```python
from build123d import *

# Parameters (mm, degrees)
F0_W     = 11.176
F0_H     = 26.5938
F1_DEPTH = 4.6482
F2_R     = 5.08
F4_DEPTH = 3.302


with BuildPart() as f1:
    # F0 (on Top) → F1 (new body)
    with BuildSketch(Plane.XY):
        Rectangle(F0_W, F0_H)
    extrude(amount=F1_DEPTH)

    # F2
    f2_edges = [f1.edges().sort_by_distance(p)[0] for p in [
        (-5.588, 13.2969, 2.3241),
        (5.588, 13.2969, 2.3241),
        (-5.588, -13.2969, 2.3241),
        (5.588, -13.2969, 2.3241),
    ]]
    fillet(f2_edges, radius=F2_R)

    # F3 (on face) → F4 (cut)
    with BuildSketch(Plane.XY):
        with BuildLine():
            Line((-4.938699, 8.085186), (-4.938699, -8.085186))
            ThreePointArc((-4.938699, -8.085186), (-3.599592, -11.318078), (-0.366699, -12.657186))
            Line((-0.366699, -12.657186), (0.366699, -12.657186))
            ThreePointArc((0.366699, -12.657186), (3.599592, -11.318078), (4.938699, -8.085186))
            Line((4.938699, -8.085186), (4.938699, 8.085186))
            ThreePointArc((4.938699, 8.085186), (3.599592, 11.318078), (0.366699, 12.657186))
            Line((0.366699, 12.657186), (-0.366699, 12.657186))
            ThreePointArc((-0.366699, 12.657186), (-3.599592, 11.318078), (-4.938699, 8.085186))
        make_face()
    extrude(amount=F4_DEPTH, mode=Mode.SUBTRACT)


solid = f1.part
```
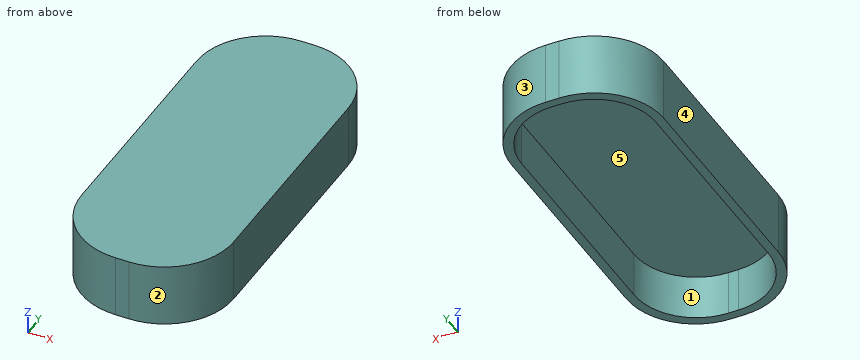
The model under review builds one solid part; all positions refer to its coordinate system, in mm. Face numbers are marked on the shaded views. A direction names the side the tool comes from. Round coordinates to 2 decimals unless told otherwise and drop trailing zeros. Order: outer loops, then holes, each group sorted by start corner. A loop starts at its lowest first (then second) coordinate and runs counter-clockwise, first axis right, second up.
(1) Tool access review of the marked faces 1 and 2: name each direction out of +Z, -Z, +X, -X, +Y, -Y from which nothing blocks a thin tool from reaching the whole face with its end or side.
Working result:
face 1: -Z
face 2: +Z, -Z, +X, -Y
(2) Take a section at B-B, the plane z = 1.05. State the section outline as (x, y) points, plus the area to 3 significant figures.
Working result:
outline: (-5.59, -8.22) arc R5.08 ccw to (-0.51, -13.3) - (0.51, -13.3) arc R5.08 ccw to (5.59, -8.22) - (5.59, 8.22) arc R5.08 ccw to (0.51, 13.3) - (-0.51, 13.3) arc R5.08 ccw to (-5.59, 8.22) - close; hole (-4.94, -8.09) arc R4.57 ccw to (-0.37, -12.66) - (0.37, -12.66) arc R4.57 ccw to (4.94, -8.09) - (4.94, 8.09) arc R4.57 ccw to (0.37, 12.66) - (-0.37, 12.66) arc R4.57 ccw to (-4.94, 8.09) - close
area: 43.0 mm2
(3) For P1, Ø1, axis at x = 3, z = 2.5, coming from the +Y side; P2, Ø5, axis at x = 0.5, y = 5.5, coming from the -Z side, all flat-tipped, find the tip position at first contact; note any pin that passes through.
Working result:
P1: stops at y = 12.89
P2: stops at z = 3.3
(4) Wall thickness on L1, parallel to X at y = 6.25, z = 0.45; L2, parallel to Z at x = 4.5, y = -9.5; L3, parallel to Y at x = 2.5, z = 0.2: over which ranges is each line inside the solid? List them lowest first.
Working result:
L1: x = -5.59 to -4.94, 4.94 to 5.59
L2: z = 3.3 to 4.65
L3: y = -12.89 to -12.13, 12.13 to 12.89
(5) Mouldability with a two-part tool opening along X and no side actions: class the marked faces 3, 4 and 5 as released by +X, released by -X, zero draft, split by the parting line, or undercut.
Working result:
face 3: released by +X
face 4: released by -X
face 5: undercut
(6) Take a section at C-C, the plane y = -4.5. State the section outline as (x, z) points.
Working result:
outline: (-5.59, 0) - (-4.94, 0) - (-4.94, 3.3) - (4.94, 3.3) - (4.94, 0) - (5.59, 0) - (5.59, 4.65) - (-5.59, 4.65) - close
(7) Take a section at A-A, the plane x = 0. State the section outline as (y, z) points, plus the area to 3 significant figures.
Working result:
outline: (-13.3, 0) - (-12.66, 0) - (-12.66, 3.3) - (12.66, 3.3) - (12.66, 0) - (13.3, 0) - (13.3, 4.65) - (-13.3, 4.65) - close
area: 40.0 mm2
